Part model, mm, in its own coordinate system. Face numbers are marked on the shaded views. A direction names the side the tool comes from. Coordinates: 2 decimals unless noted, no trailing zeros. Write each loop counter-clockwise with the first axis right and the second up, starting at its lowest first coordinate (ties: lowest second). Pieces come first, ordered by that corner, then holes. Notation, with made-up numbers: (-21, 33.5) -> (-6, 33.5) arc R26 cw to (-6, 72.5) -> close; hole circle Ø9 at (5, 61.25). An arc over 180 degrees is marked (long way). Write item = value, one per line. Start each with the question number.
Q1. Pull direction Y, two halves, no side cores. Call the marked faces 4, 5, 6 and 7: released by +Y, released by -Y, zero draft, split by the parting line, or undercut.
Q2. Tool access for the marked faces 1, 2 and 3: list every direction of +Z, -Z, +X, -X, +Y, -Y with a clear straight run to the whole face (end or side of a thin tool).
Q3. Band-saw the part on C-C, the plane x = -3. List the corners of the cut face in (y, z), plus the area to 3 significant figures.
Q4. Probe line 1 (Z direction, x = -52.5, y = -12); line 2 (X direction, y = -17, z = 26); line 3 (Y direction, x = -2.5, z = 66.5). List the from-to ranges inside material, lowest first.
Q5. Band-saw the part on B-B, the plane y = -2.5. List the corners of the cut face in (x, z), plus the area to 3 significant figures.
Q6. Pin check, flat tips, straight feed: P1, Ø20, axis at x = -16.5, y = -22.5, coming from the +Z side; P2, Ø8, axis at x = -5.5, z = 12.5, coming from the -Y side; P3, Ø4, axis at x = -43.5, y = 42.5, coming from the +Z side; P4, Ø3, axis at x = -45.5, z = 59, coming from the +Y side. Stop position of each tip, or through.
Q7. Band-saw the part on A-A, the plane y = -16.5. List the corners of the cut face in (x, z).
Q8. Band-saw the part on D-D, the plane z = 52. List the corners of the cut face in (x, y), plus the area to 3 significant figures.
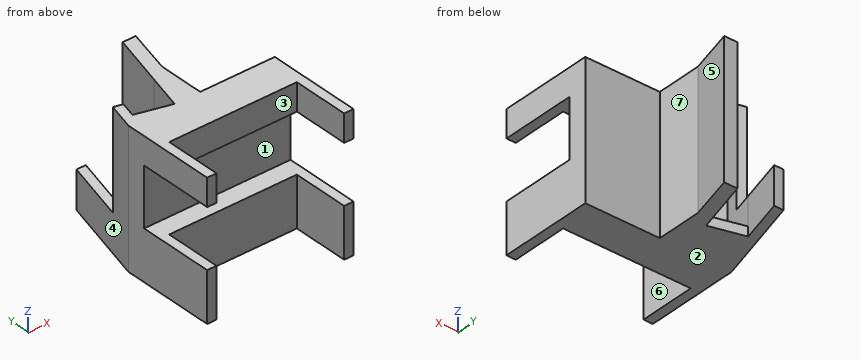
from build123d import *

# Parameters (mm, degrees)
EXTRUDE_1_DEPTH     = 72
SKETCH_2_W          = 68.186813186
SKETCH_2_H          = 31
CUT_EXTRUDE_1_DEPTH = 10
SKETCH_3_W          = 5
SKETCH_3_H          = 31
CUT_EXTRUDE_3_DEPTH = 40
SKETCH_4_W          = 5
SKETCH_4_H          = 31
CUT_EXTRUDE_4_DEPTH = 40
EXTRUDE_6_DEPTH     = 5
EXTRUDE_7_DEPTH     = 67
SKETCH_12_W         = 52
SKETCH_12_H         = 36.720454309
CUT_EXTRUDE_5_DEPTH = 5


with BuildPart() as part:
    # 草圖1 → 填料-伸長1 (new body)
    with BuildSketch(Plane.XY):
        Polygon((-56.41038016, 13.571428571), (-56.41038016, -36.428571429), (-51.41038016, -36.428571429), (-51.41038016, -6.428571429), (16.776433026, -6.428571429), (16.776433026, -36.428571429), (21.776433026, -36.428571429), (21.776433026, 13.571428571), align=None)
    extrude(amount=EXTRUDE_1_DEPTH)

    # 草圖2 → 除料-伸長1 (cut)
    with BuildSketch(Plane.XZ.offset(6.428571429)):
        with Locations((-17.316973567, 42)):
            Rectangle(SKETCH_2_W, SKETCH_2_H)
    extrude(amount=-CUT_EXTRUDE_1_DEPTH, mode=Mode.SUBTRACT)

    # 草圖3 → 除料-伸長3 (cut)
    with BuildSketch(Plane.XZ.offset(36.428571429)):
        with Locations((-53.91038016, 42)):
            Rectangle(SKETCH_3_W, SKETCH_3_H)
    extrude(amount=-CUT_EXTRUDE_3_DEPTH, mode=Mode.SUBTRACT)

    # 草圖4 → 除料-伸長4 (cut)
    with BuildSketch(Plane.XZ.offset(36.428571429)):
        with Locations((19.276433026, 42)):
            Rectangle(SKETCH_4_W, SKETCH_4_H)
    extrude(amount=-CUT_EXTRUDE_4_DEPTH, mode=Mode.SUBTRACT)

    # 草圖10 → 填料-伸長6 (add)
    with BuildSketch(Plane.XY):
        Polygon((-56.41038016, 13.571428571), (-43.469427905, 61.867719886), (-38.469427905, 61.867719886), (-44.939904033, 37.719574229), (-26.587313333, 32.802012372), (-18.799180477, 61.867719886), (-11.799180477, 61.867719886), (-18.038970236, 37.658939996), (-18.038970236, 13.571428571), align=None)
    extrude(amount=EXTRUDE_6_DEPTH)

    # 草圖11 → 填料-伸長7 (add)
    with BuildSketch(Plane.XY.offset(5)):
        Polygon((-43.469427905, 61.867719886), (-56.41038016, 13.571428571), (-31.740132733, 13.571428571), (-50.092723432, 18.488990428), (-44.939904033, 37.719574229), (-38.469427905, 61.867719886), align=None)
        Polygon((-26.587313333, 32.802012372), (-31.740132733, 13.571428571), (-18.038970236, 13.571428571), (-18.038970236, 37.658939996), (-11.799180477, 61.867719886), (-18.799180477, 61.867719886), align=None)
    extrude(amount=EXTRUDE_7_DEPTH)

    # 草圖12 → 除料-伸長5 (cut)
    with BuildSketch(Plane(origin=(-56.024458351, 15.011708372, 0), x_dir=(0, 0, 1), z_dir=(-0.965925826, 0.258819045, 0))):
        with Locations((46, 31.869139784)):
            Rectangle(SKETCH_12_W, SKETCH_12_H)
    extrude(amount=-CUT_EXTRUDE_5_DEPTH, mode=Mode.SUBTRACT)


solid = part.part
Ans:
q1.face_4 = released by +Y
q1.face_5 = undercut
q1.face_6 = zero draft
q1.face_7 = undercut
q2.face_1 = +X, -X, -Y
q2.face_2 = -Z, +X, -X, +Y, -Y
q2.face_3 = +Z, -Z, -Y
q3.outline = (-6.43, 0) -> (13.57, 0) -> (13.57, 72) -> (-6.43, 72) -> (-6.43, 57.5) -> (3.57, 57.5) -> (3.57, 26.5) -> (-6.43, 26.5) -> close
q3.area = 1,130 mm2
q4.line_1 = 0 to 26.5, 57.5 to 72
q4.line_2 = -56.41 to -51.41, 16.78 to 21.78
q4.line_3 = -6.43 to 13.57
q5.outline = (-56.41, 0) -> (21.78, 0) -> (21.78, 26.5) -> (-56.41, 26.5) -> close; (-56.41, 57.5) -> (21.78, 57.5) -> (21.78, 72) -> (-56.41, 72) -> close
q5.area = 3,210 mm2
q6.P1 = through
q6.P2 = -6.43
q6.P3 = 20
q6.P4 = 17.66
q7.outline = (-56.41, 0) -> (-51.41, 0) -> (-51.41, 26.5) -> (-56.41, 26.5) -> close; (-56.41, 57.5) -> (-51.41, 57.5) -> (-51.41, 72) -> (-56.41, 72) -> close; (16.78, 0) -> (21.78, 0) -> (21.78, 26.5) -> (16.78, 26.5) -> close; (16.78, 57.5) -> (21.78, 57.5) -> (21.78, 72) -> (16.78, 72) -> close
q8.outline = (-56.41, 3.57) -> (21.78, 3.57) -> (21.78, 13.57) -> (-18.04, 13.57) -> (-18.04, 37.66) -> (-11.8, 61.87) -> (-18.8, 61.87) -> (-31.74, 13.57) -> (-50.09, 18.49) -> (-47.86, 26.81) -> (-52.53, 28.06) -> (-56.41, 13.57) -> close
q8.area = 1,320 mm2
